Autodesk Inventor part; units mm, degrees
ref_plane "YZ Plane" through (0, 0, 0) normal (1, 0, 0) x (0, 1, 0)
ref_plane "XZ Plane" through (0, 0, 0) normal (0, 1, 0) x (-1, 0, 0)
ref_plane "XY Plane" through (0, 0, 0) normal (0, 0, 1) x (1, 0, 0)
sketch "Sketch1" plane through (0, 0, 0) normal (1, 0, 0) x (0, 1, 0)
  circle A0 centre (0, 0) radius 6.35
  dimension "d0" = 12.7
extrude "Extrusion1" add sketch "Sketch1" along normal mid plane 101.6
sketch "Sketch2" plane through (50.8, 0, 0) normal (1, 0, 0) x (0, 0, -1)
  circle A0 centre (0, 0) radius 10.16
  dimension "d3" = 20.32
extrude "Extrusion2" add sketch "Sketch2" along normal blind 3.175
sketch "Sketch3" plane through (-50.8, 0, 0) normal (-1, 0, 0) x (0, 0, 1)
  line L0 (-1.5875, 3.175) -> (-1.5875, 9.525)
  line L1 (-1.5875, 9.525) -> (1.5875, 9.525)
  line L2 (1.5875, 9.525) -> (1.5875, 3.175)
  line L3 (1.5875, 3.175) -> (-1.5875, 3.175)
  circle A0 centre (0, 0) radius 6.35
  line L4 (-1.5875, 3.175) -> (1.5875, 9.525) construction
  line L5 (-1.5875, 9.525) -> (1.5875, 3.175) construction
  point P0 (0, 6.35)
  dimension "d6" = 6.35
  dimension "d7" = 3.175
extrude "Extrusion3" cut sketch "Sketch3" against normal blind 25.4 contours L0 A0 L2 L3 | L0 L1 L2 A0 picked at (-0.1781, 4.2258)
sketch "Sketch4" plane through (-50.8, 3.175, 1.5875) normal (0, 0, -1) x (-1, 0, 0)
  point P0 (-50.8, -3.175)
properties part number "handle insert"
For this review, take the finished solid that the model builds, in its own axes (mm). A direction names the side the tool comes from. Coordinates: 2 decimals unless noted, no trailing zeros. Write each loop counter-clockwise with the first axis right and the second up, starting at its lowest first coordinate (ties: lowest second). Pieces come first, ordered by that corner, then holes. Notation, with made-up numbers: (-12.75, -8.75) -> (17.25, -8.75) arc R18 cw to (17.25, 15.25) -> close; hole circle Ø10 at (12.5, 28.25). An arc over 180 degrees is marked (long way). Write each question's results on one line, items separated by ' | '. Start each with the question number.
1) Consider section A-A (z = 0). Write out the cut boundary in (x, y) (3 decimals), plus the area to 3 significant figures.
2) Insertion check: pin 1 (1 mm diameter, centred on x = -7, y = 3, fed in from -Z); pin 2 (8 mm diameter, centred on x = -9, z = 0, fed in from -Y); pin 3 (10 mm diameter, centred on x = 40.5, y = 4.5, fed in from -Z). Each pin has a flat end and moves straight along its axis. Give the tip position at first contact, or say it passes through.
3) For faces 1 (the face through (-38, 5, 1.588)), 2 (the face through (52.365, -10.074, 1.323)), list the 3-axis set-ups (+Z, -Z, +X, -X, +Y, -Y) from which the entire face can be reached by the end or side of a thin tool; tool diameter is ignored.
4) The part is to be moulded in two halves that separate along Z. For faces 3 (the face through (-38, 3.175, 0)), 4 (the face through (-0.71, -1.38, 6.2)), 5 (the face through (50.8, -7, 0)), say which applies: +Z half, -Z half, draft (parallel to the pull), parting line (faces both ways), or undercut.
5) Consider section B-B (y = 0). Write out the cut boundary in (x, z) (3 decimals).
6) Wall thickness on L1, parallel to X at y = 8, z = 0.25 (3 decimals); L2, parallel to Y at x = 30, z = 0.5; L3, parallel to Z at x = -32.5, y = 2: over which ranges is each line inside the solid? List them lowest first. Write a range as [from, to].
7) Consider section C-C (x = 44.5). Write out the cut boundary in (y, z).
Geometry says:
1) outline: (-50.8, -6.35) -> (50.8, -6.35) -> (50.8, -10.16) -> (53.975, -10.16) -> (53.975, 10.16) -> (50.8, 10.16) -> (50.8, 6.35) -> (-25.4, 6.35) -> (-25.4, 3.175) -> (-50.8, 3.175) -> close | area: 1,270 mm^2
2) pin 1: z = -5.84 | pin 2: y = -6.35 | pin 3: z = -6.35
3) face 1: -X, +Y | face 2: +X, -X
4) face 3: undercut | face 4: parting line | face 5: draft
5) outline: (-50.8, -6.35) -> (50.8, -6.35) -> (50.8, -10.16) -> (53.975, -10.16) -> (53.975, 10.16) -> (50.8, 10.16) -> (50.8, 6.35) -> (-50.8, 6.35) -> close
6) L1: [50.8, 53.975] | L2: [-6.33, 6.33] | L3: [-6.03, 6.03]
7) outline: circle Ø12.7 at (0, 0)
